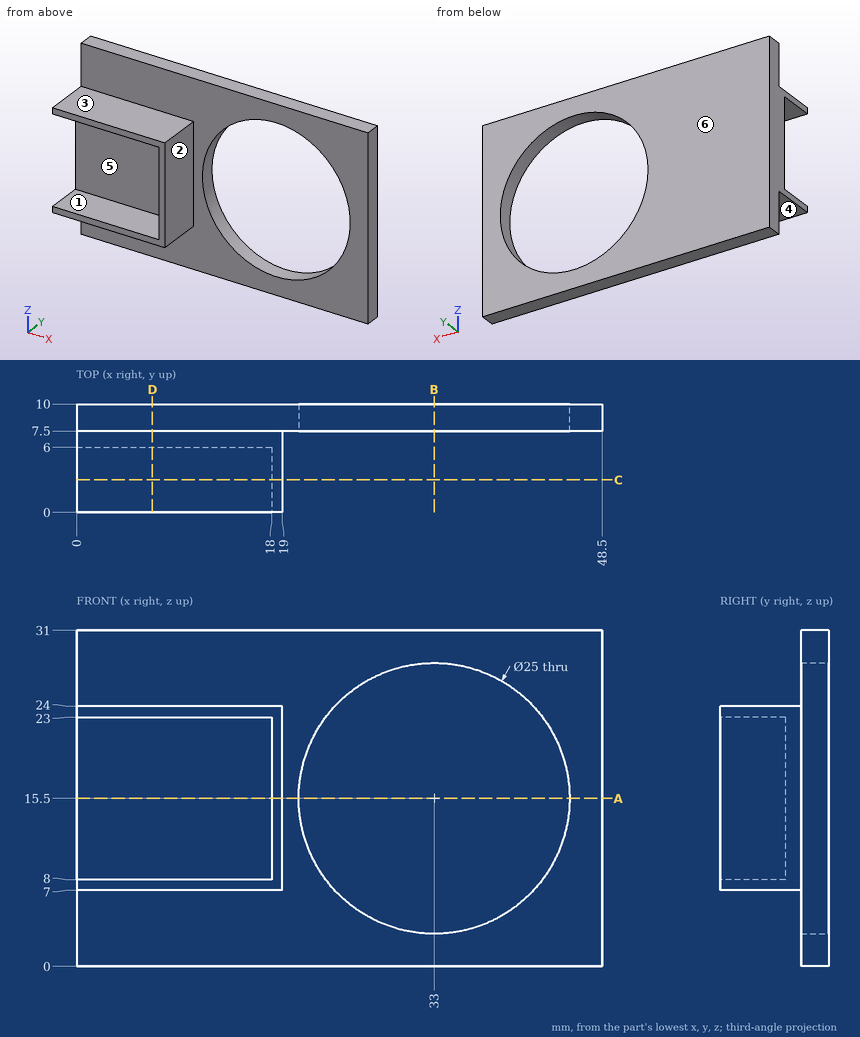
Geometry: see drawing. Coordinates: mm, zero at the bounding-box minimum. A direction names the side the tool comes from. Round coordinates to 2 decimals unless told otherwise and drop trailing zeros. Loops run counter-clockwise (first coordinate to the right, second up) from the corner with the lowest first, then second, coordinate; pieces in that order, holes last. Notation, with made-up numbers: (-7.5, -40) - (7.5, -40) arc R16 cw to (7.5, -28) - close; hole circle Ø7 at (8, -15). An arc over 180 degrees is marked (long way). Write item = value, one per line. Start each with the question number.
(1) Section query B-B, the plane x = 33. Output: boundary loops of the cut face in (y, z), plus the area to 3 significant figures.
(2) Section query C-C, the plane y = 3. Output: boundary loops of the cut face in (x, z), plus the area to 3 significant figures.
(3) Section query A-A, the plane z = 15.5. Output: boundary loops of the cut face in (x, y), plus the area to 4 significant figures.
(4) Section query D-D, the plane x = 7. Output: boundary loops of the cut face in (y, z).
(5) Ray query, line 1 along Z through (x, y) = (33, 8.1); line 2 along Z through (x, y) = (7, 2.5); line 3 along Y through (x, z) = (15.5, 15.5). Return the intervals inside material, ascending. Write a range as from..to.
(6) Pin query (flat end, axial travel): pin 1 (2 mm diameter, centred on x = 15.5, y = 5, fed in from -Z); pin 2 (1.8 mm diameter, centred on y = 2.5, z = 15, fed in from -X); pin 3 (5 mm diameter, centred on x = 10, y = 2, fed in from +Z). Return the tip coordinate at first contact, or that it passes through.
(7) Set-up query: the marked faces 1, 2 and 3. Return all of +Z, -Z, +X, -X, +Y, -Y with unobstructed straight access to the full face (end or side cutting, diameter ignored); none if empty.
(8) Pull-direction query (Z, two-part tool) for the marked faces 4, 5 and 6; classes: +Z half, -Z half, draft (parallel to the pull), parting line (faces both ways), or undercut.
Conclusion:
q1.outline = (7.5, 0) - (10, 0) - (10, 3) - (7.5, 3) - close; (7.5, 28) - (10, 28) - (10, 31) - (7.5, 31) - close
q1.area = 15.0 mm2
q2.outline = (0, 7) - (19, 7) - (19, 24) - (0, 24) - (0, 23) - (18, 23) - (18, 8) - (0, 8) - close
q2.area = 53.0 mm2
q3.outline = (0, 6) - (18, 6) - (18, 0) - (19, 0) - (19, 7.5) - (20.5, 7.5) - (20.5, 10) - (0, 10) - close; (45.5, 7.5) - (48.5, 7.5) - (48.5, 10) - (45.5, 10) - close
q3.area = 93.25 mm2
q4.outline = (0, 7) - (7.5, 7) - (7.5, 0) - (10, 0) - (10, 31) - (7.5, 31) - (7.5, 24) - (0, 24) - (0, 23) - (6, 23) - (6, 8) - (0, 8) - close
q5.line_1 = 0..3, 28..31
q5.line_2 = 7..8, 23..24
q5.line_3 = 6..10
q6.pin_1 = 7
q6.pin_2 = 18
q6.pin_3 = 24
q7.face_1 = -X, -Y
q7.face_2 = +Z, -Z, +X, -Y
q7.face_3 = +Z, +X, -X, -Y
q8.face_4 = -Z half
q8.face_5 = undercut
q8.face_6 = draft
